The figure shows three views and two pictorial views of one solid part (mm, origin at its lowest corner). Answer the questions. A direction names the side the tool comes from. Coordinates: 2 decimals unless noted, no trailing zeros. Order: outer loops, then holes, each group sorted by start corner. A loop starts at its lowest first (then second) coordinate and runs counter-clockwise, first axis right, second up. Notation, with made-up numbers: (55, 68) - (91, 68) arc R10 ccw to (91, 79) - close; hole circle Ø7 at (57, 83). An arc over 180 degrees is marked (long way). Use one line per item in the form item = value. Start each with the question number.
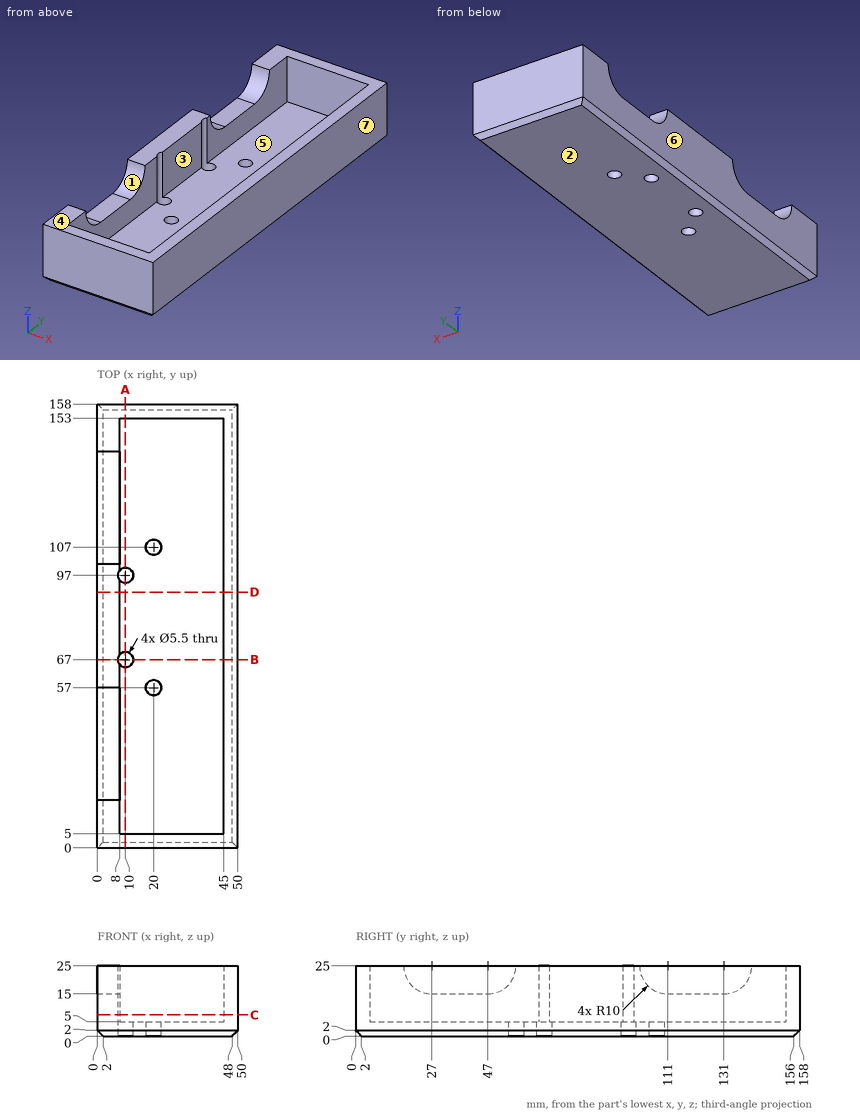
Q1. Which of the six approach directions +Z, -Z, +X, -X, +Y, -Y give full straight-line access (tool end or side, diameter ignored) to the marked faces 1, 2 and 3?
Q2. A cutting plane is placed at D-D (y = 91). Give the vertices of the cut face in (x, z).
Q3. A cutting plane is placed at B-B (y = 67). Give the vertices of the cut face in (x, z).
Q4. A cutting plane is placed at A-A (x = 10). Give the vertices of the cut face in (y, z).
Q5. Consider probe 1 along Y at (x, z) = (20, 3.7); probe 2 along X at (y, z) = (72, 9); probe 3 along Y at (x, z) = (39, 9.25). Determine where each line is inside the solid, lowest interval first.
Q6. A cutting plane is placed at C-C (z = 7.5). Give the vertices of the cut face in (x, y), then the cut area to 3 significant figures.
Q7. Given P1, Ø9, axis at x = 5, y = 32, coming from the +Z side; P2, Ø5, axis at x = 20, y = 107, coming from the +Z side, each flat-ended and moving along its own axis, determine where each tip first touches the part or whether it passes through.
Q8. For a pull along X with two mould halves and no side action, classify the marked faces 4, 5, 6 and 7 as +X half, -X half, draft (parallel to the pull), parting line (faces both ways), or undercut.
Result sheet:
q1.face_1 = +Z, -X
q1.face_2 = -Z, +X, -X, +Y, -Y
q1.face_3 = +Z
q2.outline = (0, 2) - (2, 0) - (48, 0) - (50, 2) - (50, 25) - (45, 25) - (45, 5) - (8, 5) - (8, 25) - (0, 25) - close
q3.outline = (0, 2) - (2, 0) - (7.25, 0) - (7.25, 25) - (0, 25) - close; (12.75, 0) - (48, 0) - (50, 2) - (50, 25) - (45, 25) - (45, 5) - (12.75, 5) - close
q4.outline = (0, 2) - (2, 0) - (64.25, 0) - (64.25, 5) - (5, 5) - (5, 25) - (0, 25) - close; (69.75, 0) - (94.25, 0) - (94.25, 5) - (69.75, 5) - close; (99.75, 0) - (156, 0) - (158, 2) - (158, 25) - (153, 25) - (153, 5) - (99.75, 5) - close
q5.probe_1 = 0 to 54.25, 59.75 to 104.25, 109.75 to 158
q5.probe_2 = 0 to 8, 45 to 50
q5.probe_3 = 0 to 5, 153 to 158
q6.outline = (0, 0) - (50, 0) - (50, 158) - (0, 158) - close; hole (8, 5) - (45, 5) - (45, 153) - (8, 153) - (8, 98.89) arc R2.75 ccw to (8, 95.11) - (8, 68.89) arc R2.75 ccw to (8, 65.11) - close
q6.area = 2,420 mm^2
q7.P1 = 15
q7.P2 = through
q8.face_4 = draft
q8.face_5 = undercut
q8.face_6 = -X half
q8.face_7 = +X half
